The model under review builds one solid part; all positions refer to its coordinate system, in mm. A direction names the side the tool comes from. Coordinates: 2 decimals unless noted, no trailing zeros. Write each loop counter-clockwise with the first axis right and the second up, starting at its lowest first coordinate (ties: lowest second). Pieces come first, ordered by that corner, then holes. Notation, with made-up numbers: M 0,60.5 L 12,60.5 A23 ccw 12,75.5 Z; hole C 67,-6.75 d2. An arc over 180 degrees is marked long. Answer as CSV lines item,"result". Start each with the question number.
from build123d import *

# Parameters (mm, degrees)
SKETCH1_R           = 1.25
BOSS_EXTRUDE1_DEPTH = 12.25
CUT_EXTRUDE1_REACH  = 94.464
SKETCH2_R           = 3
FILLET1_R           = 1.25
CUT_EXTRUDE2_REACH  = 94.757


with BuildPart() as part:
    # Sketch1 → Boss-Extrude1 (new body)
    with BuildSketch(Plane.XY):
        with BuildLine():
            Line((0.25, -3.240370349), (0.25, -41.740370349))
            Line((0.25, -41.740370349), (8.25, -85.075157412))
            ThreePointArc((8.25, -85.075157412), (10.208936196, -88.421482437), (13.855284626, -89.740370349))
            Line((13.855284626, -89.740370349), (18.855284626, -89.740370349))
            Line((18.855284626, -89.740370349), (18.855284626, -86.740370349))
            Line((18.855284626, -86.740370349), (13.855284626, -86.740370349))
            ThreePointArc((13.855284626, -86.740370349), (12.129255683, -86.116622764), (11.200712952, -84.533573379))
            Line((11.200712952, -84.533573379), (3.25, -41.740370349))
            Line((3.25, -41.740370349), (3.25, 0))
            ThreePointArc((3.25, 0), (-2.384848004, 2.207940217), (0.25, -3.240370349))
        make_face()
        Circle(SKETCH1_R, mode=Mode.SUBTRACT)
    extrude(amount=BOSS_EXTRUDE1_DEPTH)

    # Sketch2 → Cut-Extrude1 (cut, up to next)
    with BuildSketch(Plane.ZY.offset(-0.25), mode=Mode.PRIVATE) as cut_extrude1_sk1:
        with Locations(Location((6.125, -31, 0), (0, 0, 270))):
            Circle(SKETCH2_R)
    cut_extrude1_tool1 = extrude(cut_extrude1_sk1.sketch, amount=-CUT_EXTRUDE1_REACH, mode=Mode.PRIVATE) & part.part
    add(cut_extrude1_tool1.solids().sort_by_distance((0.25, -31, 6.125))[0], mode=Mode.SUBTRACT)

    # Fillet1
    fillet1_edges = [part.edges().sort_by_distance(p)[0] for p in [
        (0.25, -28, 6.125),
        (3.25, -28, 6.125),
    ]]
    fillet(fillet1_edges, radius=FILLET1_R)

    # Sketch4 → Cut-Extrude2 (cut, up to next)
    with BuildSketch(Plane(origin=(0, -86.740370349, 0), x_dir=(1, 0, 0), z_dir=(0, 1, 0)), mode=Mode.PRIVATE) as cut_extrude2_sk1:
        with BuildLine():
            Line((18.855284626, 0), (18.855284626, -12.25))
            ThreePointArc((18.855284626, -12.25), (17.547778007, -6.125), (18.855284626, 0))
        make_face()
    cut_extrude2_tool1 = extrude(cut_extrude2_sk1.sketch, amount=-CUT_EXTRUDE2_REACH, mode=Mode.PRIVATE) & part.part
    add(cut_extrude2_tool1.solids().sort_by_distance((18.330278, -86.74037, 6.125))[0], mode=Mode.SUBTRACT)


solid = part.part
1) Clearance check with flat-ended pins moving along their axes: pin 1 Ø5 at (y, z) = (-31, 6.125) entering from -X; pin 2 Ø1.5 at (y, z) = (-47.5, 2) entering from +X; pin 3 Ø5.5 at (x, z) = (16.5, 8) entering from +Y; pin 4 Ø4 at (y, z) = (-6.5, 5) entering from +X. State where each tip first meets the part, or that it passes through.
2) Take a section at D-D on y = -68. Give the boundary of the cut face in (x, z), and give its area (3 significant figures).
3) Take a section at C-C on y = -57. Give the boundary of the cut face in (x, z).
4) To check wall thickness, follow line 1 (Y direction, x = 0, z = 7); line 2 (Z direction, x = 1.65, y = -31) (3 decimals); line 3 (X direction, y = -20, z = 2.25). State the ranges of each line that lie inside material, in increasing order. Write a range as [from, to].
5) Mouldability with a two-part tool opening along Z and no side actions: class faces 4 (the cylindrical face through (17.55, -88.22, 6.21)), 5 (the flat face through (2, -43, 0)), 6 (the flat face through (16, -89.74, 6)) as +Z half, -Z half, draft (parallel to the pull), parting line (faces both ways), or undercut.
6) Tool access review of faces 1 (the flat face through (3.25, -21, 6)), 2 (the flat face through (0.25, -22, 6)), 3 (the flat face through (2, -43, 12.25)): name each direction out of +Z, -Z, +X, -X, +Y, -Y from which nothing blocks a thin tool from reaching the whole face with its end or side.
7) Take a section at B-B on z = 4.5. Give the number of separate pieces and of enclosed holes in the cut face, and give its area (3 significant figures).
8) Take a section at A-A on y = -31. Give the boundary of the cut face in (x, z) (3 decimals).
Results:
1,pin 1,"passes through"
1,pin 2,"stops at x = 4.46"
1,pin 3,"stops at y = -86.74"
1,pin 4,"stops at x = 3.25"
2,outline,"M 5.1,0 L 8.13,0 L 8.13,12.25 L 5.1,12.25 Z"
2,area,"37.1 mm²"
3,outline,"M 3.07,0 L 6.09,0 L 6.09,12.25 L 3.07,12.25 Z"
4,line 1,"y = [-3.25, -1.25], [1.25, 3.25]"
4,line 2,"z = [0, 3.125], [9.125, 12.25]"
4,line 3,"x = [0.25, 3.25]"
5,face 4,"undercut"
5,face 5,"-Z half"
5,face 6,"draft"
6,face 1,"+Z, -Z, +X, +Y"
6,face 2,"+Z, -Z, -X, -Y"
6,face 3,"+Z, +X, -X, +Y, -Y"
7,separate pieces,"2"
7,enclosed holes,"1"
7,area,"288 mm²"
8,outline,"M 0.25,0 L 3.25,0 L 3.25,1.875 A1.25 ccw 2,3.125 L 1.5,3.125 A1.25 ccw 0.25,1.875 Z; M 0.25,10.375 A1.25 ccw 1.5,9.125 L 2,9.125 A1.25 ccw 3.25,10.375 L 3.25,12.25 L 0.25,12.25 Z"
